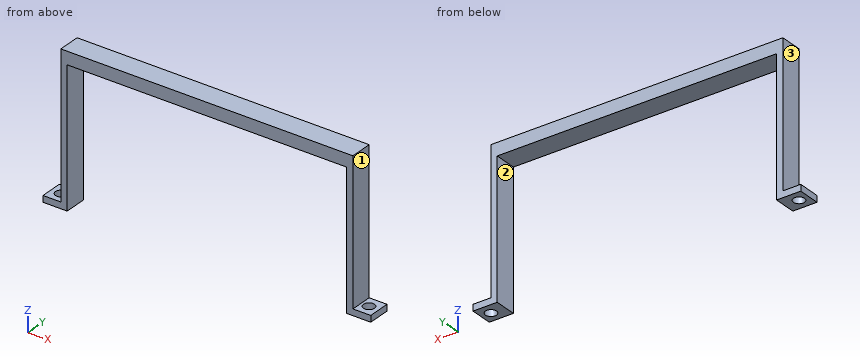
Autodesk Inventor part; units mm, degrees
ref_plane "YZ Plane" through (0, 0, 0) normal (1, 0, 0) x (0, 1, 0)
ref_plane "XZ Plane" through (0, 0, 0) normal (0, 1, 0) x (-1, 0, 0)
ref_plane "XY Plane" through (0, 0, 0) normal (0, 0, 1) x (1, 0, 0)
sketch "Sketch1" plane through (0, 0, 0) normal (0, 0, 1) x (1, 0, 0)
  line L0 (0, 0) -> (88, 0)
  line L1 (88, 0) -> (88, 7)
  line L2 (88, 7) -> (0, 7)
  line L3 (0, 7) -> (0, 0)
  dimension "d0" = 88
  dimension "d1" = 7
extrude "Extrusion1" add sketch "Sketch1" along normal blind 4
sketch "Sketch2" plane through (0, 0, 0) normal (0, 0, -1) x (-1, 0, 0)
  line L0 (0, 0) -> (-88, 0)
  line L1 (0, 7) -> (0, 0)
  line L2 (-88, 7) -> (0, 7)
  line L3 (-88, 0) -> (-88, 7)
  line L4 (0, 0) -> (2, 0)
  line L5 (2, 0) -> (2, 7)
  line L6 (2, 7) -> (0, 7)
  line L7 (0, 7) -> (0, 0)
  line L8 (-88, 7) -> (-90, 7)
  line L9 (-90, 7) -> (-90, 0)
  line L10 (-90, 0) -> (-88, 0)
  line L11 (-88, 0) -> (-88, 7)
  dimension "d4" = 2
  dimension "d5" = 2
extrude "Extrusion2" add sketch "Sketch2" along normal blind 41 contours L1 L6 L5 L4 | L10 L9 L8 L3
extrude "Extrusion3" add sketch "Sketch2" against normal blind 4 contours L1 L6 L5 L4 | L10 L9 L8 L3
sketch "Sketch3" plane through (0, 0, -41) normal (0, 0, -1) x (-1, 0, 0)
  line L0 (-88, 7) -> (-90, 7)
  line L1 (-90, 7) -> (-90, 0)
  line L2 (-90, 0) -> (-88, 0)
  line L3 (-88, 0) -> (-88, 7)
  line L4 (2, 0) -> (2, 7)
  line L5 (0, 0) -> (2, 0)
  line L6 (2, 0) -> (2, 7)
  line L7 (2, 7) -> (0, 7)
  line L8 (0, 7) -> (0, 0)
  line L9 (-88, 0) -> (-95.62, 0)
  line L10 (-95.62, 0) -> (-95.62, 7)
  line L11 (-95.62, 7) -> (-88, 7)
  line L12 (-88, 7) -> (-88, 0)
  circle A0 centre (-92.5085, 3.5) radius 1.75
  line L13 (0, 7) -> (7.62, 7)
  line L14 (7.62, 7) -> (7.62, 0)
  line L15 (7.62, 0) -> (0, 0)
  line L16 (0, 0) -> (0, 7)
  circle A1 centre (4.5085, 3.5) radius 1.75
  dimension "d10" = 3.5
  dimension "d12" = 3.5
  dimension "d17" = 7.62
  dimension "d18" = 7.62
  dimension "d21" = 97.017
extrude "Extrusion4" add sketch "Sketch3" along normal blind 2
Can you work these out from the model? Positions are in its coordinate system, mm. Face numbers are marked on the shaded views. Round coordinates to 2 decimals unless told otherwise and drop trailing zeros. Loops run counter-clockwise (first coordinate to the right, second up) from the corner with the lowest first, then second, coordinate; pieces in that order, holes last. Notation, with made-up numbers: (-18.75, 32.25) - (-10.75, 32.25) arc R23 cw to (-10.75, 48.25) - close; hole circle Ø11 at (-33.5, 46). An arc over 180 degrees is marked (long way). Write item = value, one per line. Start each with the question number.
(1) If we section it at B-B (z = -14.5): Please give me the cut outline in (x, y).
(2) If we mould it in two halves opening along X, with no side actions, what happens to the marked faces 1, 2 and 3? For each: released by +X, released by -X, zero draft, split by the parting line, or undercut.
(3) If we section it at C-C (x = 21): Please give me the cut outline in (y, z), and give its area (3 significant figures).
(4) If we section it at A-A (y = 3.5): Please give me the cut outline in (x, z).
(5) For P1, Ø1.7, axis at x = -4.5, y = 2, coming from the +Z side; P2, Ø3.5, axis at y = 4, z = -21.5, coming from the -X side; P3, Ø3.5, axis at x = 43, y = 4, coming from the -Z side, each with a flat end and sliding along its axis, tell me the tip position at first contact or that it passes through.
(6) If I drill on probe 1 along X at (y, z) = (6, -2); probe 2 along Z at (x, y) = (63, 0.5), over which ranges is the centre line in solid material (lowest first)? Write a range as [from, to].
Ans:
q1.outline = (-2, 0) - (0, 0) - (0, 7) - (-2, 7) - close; (88, 0) - (90, 0) - (90, 7) - (88, 7) - close
q2.face_1 = released by +X
q2.face_2 = undercut
q2.face_3 = released by -X
q3.outline = (0, 0) - (7, 0) - (7, 4) - (0, 4) - close
q3.area = 28.0 mm²
q4.outline = (-7.62, -43) - (-6.26, -43) - (-6.26, -41) - (-7.62, -41) - close; (-2.76, -43) - (0, -43) - (0, 0) - (88, 0) - (88, -43) - (90.76, -43) - (90.76, -41) - (90, -41) - (90, 4) - (-2, 4) - (-2, -41) - (-2.76, -41) - close; (94.26, -43) - (95.62, -43) - (95.62, -41) - (94.26, -41) - close
q5.P1 = -41
q5.P2 = -2
q5.P3 = 0
q6.probe_1 = [-2, 0], [88, 90]
q6.probe_2 = [0, 4]
